Work out the finished part from the listing and answer in its coordinate system (mm). A direction names the side the tool comes from. Round coordinates to 2 decimals unless told otherwise and drop trailing zeros. Loops run counter-clockwise (first coordinate to the right, second up) from the corner with the lowest first, then second, coordinate; pieces in that order, holes last. Notation, with made-up numbers: (60, 50.25) - (86, 50.25) arc R7 cw to (86, 54.25) - close; hole circle Ø2 at (70, 21). An arc over 180 degrees is marked (long way). Answer as CSV lines item,"result". Start each with the question number.
Q1. Section B-B on y = -8 is taken. Write down the section's boundary in (x, z), then the cut area to 3 significant figures.
Q2. Straight lines are drawn through the part: L1, parallel to Y at x = 0, z = -0.5; L2, parallel to X at y = 2, z = 0.6; L3, parallel to Y at x = -14, z = 0.3. For each, find the intervals that lie inside material, in ascending order. Write a range as [from, to].
Q3. Section C-C on x = 0 is taken. Write down the section's boundary in (y, z).
Q4. Section A-A on z = 0.8 is taken. Write down the section's boundary in (x, y), then the cut area to 3 significant figures.
Q5. For faces 4 (the face through (-18, 2, 0)), 5 (the face through (0, 15.5, 1)), 6 (the face through (0, 17, 1)), 7 (the face through (0, -17, 1)), determine the directions among +Z, -Z, +X, -X, +Y, -Y from which every point of the face is accessible in a straight line to the end or side of a thin tool.
Q6. Section D-D on y = -0.5 is taken. Write down the section's boundary in (x, z), then the cut area to 3 significant figures.
Q7. Each of these flat-tipped pins is pushed along its axis until it touches: pin 1 Ø0.9 at (y, z) = (5, 2) entering from +X; pin 2 Ø1 at (x, z) = (-7.5, 1) entering from -Y; pin 3 Ø0.9 at (y, z) = (-3, 1) entering from -X. Where does it stop, or does it pass through?
Q8. The mould has two halves that part along Z. Classify faces 1 (the face through (19.199, 1.801, -1.215)), 2 (the face through (-16.5, -1, 2)), 3 (the face through (0.23, -17.51, 2.56)): +Z half, -Z half, draft (parallel to the pull), parting line (faces both ways), or undercut.
```python
from build123d import *

# Parameters (mm, degrees)
F0_W        = 33
F0_H        = 34
F0_W_2      = 30
F0_H_2      = 31
F1_DEPTH    = 3
F2_W        = 39
F2_H        = 43
F3_DEPTH    = 1.5
F4_D        = 3.2
F5_T1_DEPTH = 44
F5_T3_DEPTH = 48
F7_DEPTH    = 16.5
F8_D        = 12
F9_D        = 13


# Not quite as in the source:
# - a fillet or chamfer that OpenCascade refuses, or shapes differently, is made with other operations: its cross-section is extruded or revolved along the edge and cut away or added


with BuildPart() as f1:
    # F0 (on Top) → F1 (new body)
    with BuildSketch(Plane.XY):
        Rectangle(F0_W, F0_H)
        Rectangle(F0_W_2, F0_H_2, mode=Mode.SUBTRACT)
    extrude(amount=F1_DEPTH)

    # F2 (on Top) → F3 (join)
    with BuildSketch(Plane.XY):
        with Locations((0, 1.5)):
            Rectangle(F2_W, F2_H)
    extrude(amount=-F3_DEPTH)

    # F4 (through all)
    with Locations(Plane.XY):
        with Locations((0, 20.5)):
            Hole(F4_D / 2)

    # F5: fillet of radius 1 on 4 edges, made by hand

    # F5_s2 → F5_t1 (cut)
    with BuildSketch(Plane.YZ.offset(-22)):
        with BuildLine():
            ThreePointArc((23, -0.5), (22.7071067812, -1.2071067812), (22, -1.5))
            Line((22, -1.5), (23, -1.5))
            Line((23, -1.5), (23, -0.5))
        make_face()
        with BuildLine():
            ThreePointArc((-20, -0.5), (-19.7071067812, -1.2071067812), (-19, -1.5))
            Line((-19, -1.5), (-20, -1.5))
            Line((-20, -1.5), (-20, -0.5))
        make_face()
    extrude(amount=F5_T1_DEPTH, mode=Mode.SUBTRACT)

    # F5_s4 → F5_t3 (cut)
    with BuildSketch(Plane.XZ.offset(-25.5)):
        with BuildLine():
            ThreePointArc((-19.5, -0.5), (-19.2071067812, -1.2071067812), (-18.5, -1.5))
            Line((-18.5, -1.5), (-19.5, -1.5))
            Line((-19.5, -1.5), (-19.5, -0.5))
        make_face()
        with BuildLine():
            ThreePointArc((18.5, -1.5), (19.2071067812, -1.2071067812), (19.5, -0.5))
            Line((19.5, -0.5), (19.5, -1.5))
            Line((19.5, -1.5), (18.5, -1.5))
        make_face()
    extrude(amount=F5_T3_DEPTH, mode=Mode.SUBTRACT)

    # F6 (on Right) → F7 (join, symmetric)
    with BuildSketch(Plane.YZ):
        Polygon((-17, 3), (-18, 3), (-17, 2.1), align=None)
    extrude(amount=F7_DEPTH, both=True)

    # F8 (through all)
    with Locations(Plane.XY):
        with Locations((0, 8.5)):
            Hole(F8_D / 2)

    # F9 (through all)
    with Locations(Plane.XY):
        with Locations((0, -8)):
            Hole(F9_D / 2)


solid = f1.part
```
Findings:
1,outline,"(-19.5, -0.5) arc R1 ccw to (-18.5, -1.5) - (-6.5, -1.5) - (-6.5, 0) - (-15, 0) - (-15, 3) - (-16.5, 3) - (-16.5, 0) - (-19.5, 0) - close; (6.5, -1.5) - (18.5, -1.5) arc R1 ccw to (19.5, -0.5) - (19.5, 0) - (16.5, 0) - (16.5, 3) - (15, 3) - (15, 0) - (6.5, 0) - close"
1,area,"47.6 mm^2"
2,L1,"y = [-20, -14.5], [-1.5, 2.5], [14.5, 18.9], [22.1, 23]"
2,L2,"x = [-16.5, -15], [15, 16.5]"
2,L3,"y = [-17, -15.5], [15.5, 17]"
3,outline,"(-20, -0.5) arc R1 ccw to (-19, -1.5) - (-14.5, -1.5) - (-14.5, 0) - (-15.5, 0) - (-15.5, 3) - (-18, 3) - (-17, 2.1) - (-17, 0) - (-20, 0) - close; (-1.5, -1.5) - (2.5, -1.5) - (2.5, 0) - (-1.5, 0) - close; (14.5, -1.5) - (18.9, -1.5) - (18.9, 0) - (17, 0) - (17, 3) - (15.5, 3) - (15.5, 0) - (14.5, 0) - close; (22.1, -1.49) arc R1 ccw to (23, -0.5) - (23, 0) - (22.1, 0) - close"
4,outline,"(-16.5, -17) - (16.5, -17) - (16.5, 17) - (-16.5, 17) - close; hole (-15, -15.5) - (15, -15.5) - (15, 15.5) - (-15, 15.5) - close"
4,area,"192 mm^2"
5,face 4,"none"
5,face 5,"+Z"
5,face 6,"+Z, +X, -X, +Y"
5,face 7,"+X, -X, -Y"
6,outline,"(-19.5, -0.5) arc R1 ccw to (-18.5, -1.5) - (18.5, -1.5) arc R1 ccw to (19.5, -0.5) - (19.5, 0) - (16.5, 0) - (16.5, 3) - (15, 3) - (15, 0) - (-15, 0) - (-15, 3) - (-16.5, 3) - (-16.5, 0) - (-19.5, 0) - close"
6,area,"67.1 mm^2"
7,pin 1,"stops at x = 16.5"
7,pin 2,"stops at y = -17"
7,pin 3,"stops at x = -16.5"
8,face 1,"-Z half"
8,face 2,"draft"
8,face 3,"undercut"
